Job drawing, mm, ordinate dimensions from the low corner. One solid piece. A direction names the side the tool comes from. Give positions to 0.01 mm unless a question says otherwise; leave off trailing zeros. Order: outer loops, then holes, each group sorted by start corner. A loop starts at its lowest first (then second) coordinate and runs counter-clockwise, first axis right, second up.
1. Slice it at A-A on x = 2.75. List the corners of the cut face in (y, z).
2. Drop flat-ended pins along their axis: pin 1 Ø3 at (y, z) = (2, 1.5) entering from -X; pin 2 Ø0.6 at (y, z) = (2, 5.5) entering from -X. Give the stop position or say it passes through.
3. Slice it at D-D on y = 1.35. List the corners of the cut face in (x, z), and give its area (3 significant figures).
4. Which spindle directions (+Z, -Z, +X, -X, +Y, -Y) get a long thin tool onto all of the face, cutting with end or side? Do the marked faces 1 and 2. Say none if no direction does.
5. Probe line 1 (Z direction, x = 3.9, y = 2.7); line 2 (Z direction, x = 0.7, y = 3.05); line 3 (Y direction, x = 2.6, z = 2.45). List the from-to ranges inside material, lowest first.
6. Slice it at C-C on z = 2.55. List the corners of the cut face in (x, y).
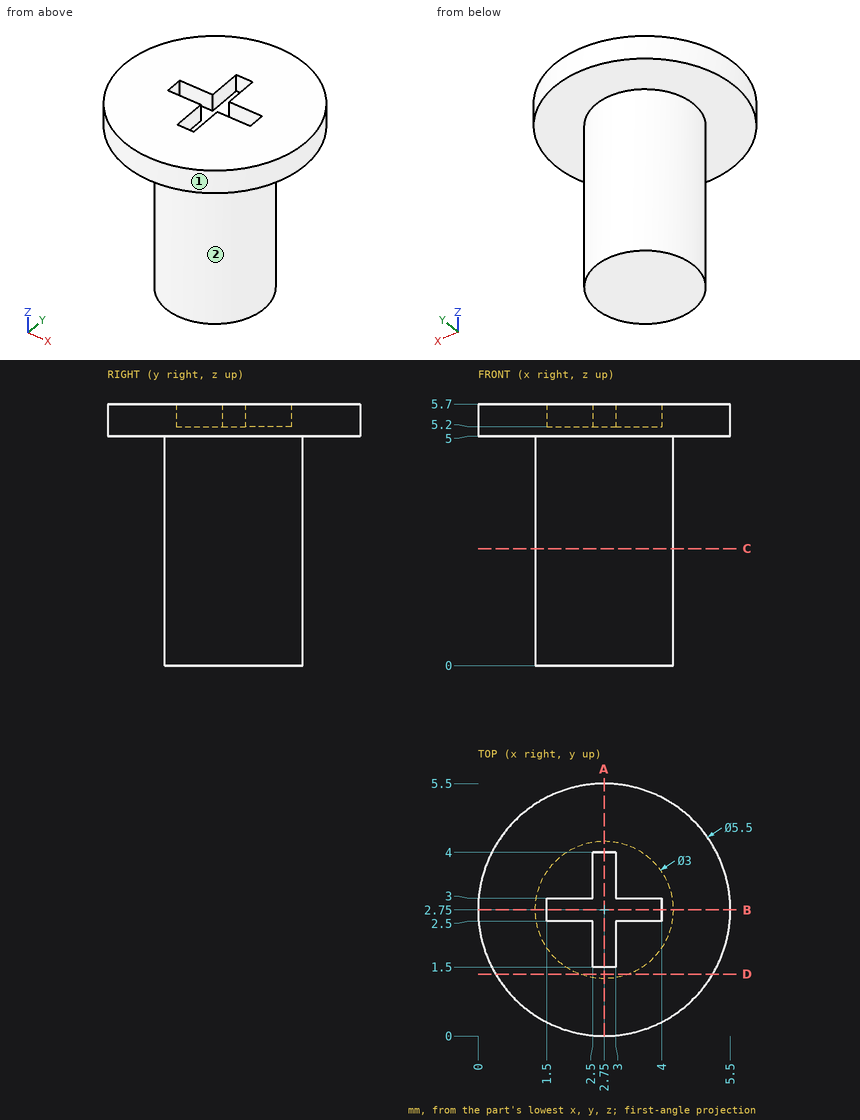
Data:
1. outline: (0, 5) - (1.25, 5) - (1.25, 0) - (4.25, 0) - (4.25, 5) - (5.5, 5) - (5.5, 5.7) - (4, 5.7) - (4, 5.2) - (1.5, 5.2) - (1.5, 5.7) - (0, 5.7) - close
2. pin 1: stops at x = 1.25
2. pin 2: stops at x = 0.04
3. outline: (0.38, 5) - (2.21, 5) - (2.21, 0) - (3.29, 0) - (3.29, 5) - (5.12, 5) - (5.12, 5.7) - (0.38, 5.7) - close
3. area: 8.70 mm2
4. face 1: +Z, -Z
4. face 2: -Z
5. line 1: z = 0 to 5.2
5. line 2: z = 5 to 5.7
5. line 3: y = 1.26 to 4.24
6. outline: circle Ø3 at (2.75, 2.75)
